from build123d import *

# Parameters (mm, degrees)
F0_W     = 100
F0_H     = 70
F1_DEPTH = 107
F2_R     = 37.5
F3_DEPTH = 61.2
F4_R     = 14.4000008702
F5_DEPTH = 131.201
F6_SIZE  = 5


with BuildPart() as f1:
    # F0 (on Front) → F1 (new body)
    with BuildSketch(Plane.XZ):
        with Locations((50, 35)):
            Rectangle(F0_W, F0_H)
    extrude(amount=F1_DEPTH)

    # F2 (on face) → F3 (join)
    with BuildSketch(Plane.XY.offset(70)):
        with Locations((50, -57)):
            Circle(F2_R)
    extrude(amount=F3_DEPTH)

    # F4 (on face) → F5 (cut, through all)
    with BuildSketch(Plane.XY.offset(131.2)):
        with Locations((50, -57)):
            Circle(F4_R)
    extrude(amount=-F5_DEPTH, mode=Mode.SUBTRACT)

    # F6
    f6_edges = [f1.edges().sort_by_distance(p)[0] for p in [
        (12.5, -57, 131.2),
        (35.599999, -57, 131.2),
        (35.599999, -57, 0),
    ]]
    chamfer(f6_edges, length=F6_SIZE)


solid = f1.part
Model file for the job. Use its own axes, mm. A direction names the side the tool comes from. Give positions to 0.01 mm unless a question says otherwise; leave off trailing zeros. Order: outer loops, then holes, each group sorted by start corner. A loop starts at its lowest first (then second) coordinate and runs counter-clockwise, first axis right, second up. Notation, with made-up numbers: (-21.5, 52.25) - (-8.5, 52.25) arc R23 ccw to (-8.5, 77.25) - close; hole circle Ø9 at (-25.5, 40). An arc over 180 degrees is marked (long way). Write item = value, one per line. Start each with the question number.
1. Drop flat-ended pins along their axis: P1, Ø3, axis at x = 80, z = 75, coming from the -Y side; P2, Ø4, axis at x = 21, y = -79.5, coming from the -Z side; P3, Ø4, axis at y = -73.5, z = 117.5, coming from the -X side; P4, Ø6, axis at x = 50, z = 77, coming from the -Y side. Give the stop position or say it passes through.
2. Cut at A-A, the plane x = 50. List the corners of the cut face in (y, z).
3. Cut at C-C, the plane z = 115. List the corners of the cut face in (x, y).
4. Two-plate mould, pull along Y, no slides. Class faces 3 (the flat face through (100, -53, 35)), 4 (the conical face through (81.231, -47.165, 130.957)), 5 (the conical face through (63.526, -62.608, 4.757)), 6 (the flat face through (49, -107, 35)): pulls with the +Y half, pulls with the -Y half, needs draft (parallel to the pull), parting line crosses it, or undercut.
5. Probe line 1 along Y through (x, z) = (50, 77); line 2 along Y through (x, z) = (50, 44); line 3 along Z through (x, y) = (32, -92.5). List the from-to ranges inside material, lowest first.
6. Cut at B-B, the plane y = -57. List the corners of the cut face in (x, z), and give its area (3 significant figures).
7. Cut at D-D, the plane y = -11. List the corners of the cut face in (x, z), and give its area (3 significant figures).
8. Which spindle directions (+Z, -Z, +X, -X, +Y, -Y) get a long thin tool onto all of the face, cutting with end or side? Do faces 1 (the flat face through (49, -17, 70)), 2 (the flat face through (0, -53, 35)). Say none if no direction does.
Taken from the geometry:
q1.P1 = -81.37
q1.P2 = 0
q1.P3 = 15.42
q1.P4 = -94.5
q2.outline = (-107, 0) - (-76.4, 0) - (-71.4, 5) - (-71.4, 126.2) - (-76.4, 131.2) - (-89.5, 131.2) - (-94.5, 126.2) - (-94.5, 70) - (-107, 70) - close; (-42.6, 5) - (-37.6, 0) - (0, 0) - (0, 70) - (-19.5, 70) - (-19.5, 126.2) - (-24.5, 131.2) - (-37.6, 131.2) - (-42.6, 126.2) - close
q3.outline = circle Ø75 at (50, -57); hole circle Ø28.8 at (50, -57)
q4.face_3 = needs draft
q4.face_4 = parting line crosses it
q4.face_5 = undercut
q4.face_6 = pulls with the -Y half
q5.line_1 = -94.5 to -71.4, -42.6 to -19.5
q5.line_2 = -107 to -71.4, -42.6 to 0
q5.line_3 = 0 to 70
q6.outline = (0, 0) - (30.6, 0) - (35.6, 5) - (35.6, 126.2) - (30.6, 131.2) - (17.5, 131.2) - (12.5, 126.2) - (12.5, 70) - (0, 70) - close; (64.4, 5) - (69.4, 0) - (100, 0) - (100, 70) - (87.5, 70) - (87.5, 126.2) - (82.5, 131.2) - (69.4, 131.2) - (64.4, 126.2) - close
q6.area = 7,740 mm²
q7.outline = (0, 0) - (100, 0) - (100, 70) - (0, 70) - close
q7.area = 7,000 mm²
q8.face_1 = +Z
q8.face_2 = +Z, -Z, -X, +Y, -Y
